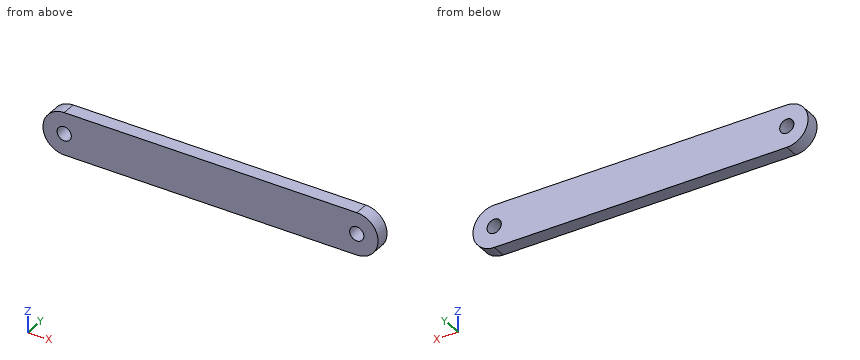
```python
from build123d import *

# Parameters (mm, degrees)
SKETCH1_R           = 2.4
BOSS_EXTRUDE1_DEPTH = 5
SCALE1_SCALE        = 0.8
SKETCH2_R           = 2
CUT_EXTRUDE1_DEPTH  = 48.792424581


with BuildPart() as part:
    # Sketch1 → Boss-Extrude1 (new body)
    with BuildSketch(Plane(origin=(0, 0, 0), x_dir=(1, 0, 0), z_dir=(0, 1, 0))):
        with BuildLine():
            Line((-51.5565916, 7.5), (51.5565916, 7.5))
            ThreePointArc((51.5565916, 7.5), (59.0565916, 0), (51.5565916, -7.5))
            Line((51.5565916, -7.5), (-51.5565916, -7.5))
            ThreePointArc((-51.5565916, -7.5), (-59.0565916, 0), (-51.5565916, 7.5))
        make_face()
        with Locations(Location((-51.5565916, 0, 0), (0, 0, 270))):
            Circle(SKETCH1_R, mode=Mode.SUBTRACT)
        with Locations(Location((51.5565916, 0, 0), (0, 0, 270))):
            Circle(SKETCH1_R, mode=Mode.SUBTRACT)
    extrude(amount=BOSS_EXTRUDE1_DEPTH)


with BuildPart() as part_1:
    # Scale1: scaled about (0, 2.5, 0)
    add(part.part.scale(SCALE1_SCALE).moved(Location((0, 0.5, 0))))

    # Sketch2 → Cut-Extrude1 (cut, through all)
    with BuildSketch(Plane(origin=(0, 4.5, 0), x_dir=(1, 0, 0), z_dir=(0, 1, 0))):
        with Locations(Location((-41.24527328, 0, 0), (0, 0, 270))):
            Circle(SKETCH2_R)
        with Locations(Location((41.24527328, 0, 0), (0, 0, 270))):
            Circle(SKETCH2_R)
    extrude(amount=-CUT_EXTRUDE1_DEPTH, mode=Mode.SUBTRACT)


solid = part_1.part
```
Design review of the part built by this model. Coordinates are the model's own, in mm. Round coordinates to 2 decimals unless told otherwise and drop trailing zeros. Order: outer loops, then holes, each group sorted by start corner. A loop starts at its lowest first (then second) coordinate and runs counter-clockwise, first axis right, second up. Notation, with made-up numbers: (49.25, -32) - (84.25, -32) arc R26 cw to (84.25, -16) - close; hole circle Ø4 at (3, -27). An arc over 180 degrees is marked (long way). Return JSON: item names as keys, results as strings.
Q1. Consider section B-B on y = 1.1. Write out the cut boundary in (x, z), plus the area to 3 significant figures.
Computed values:
{"outline": "(-41.25, -6) - (41.25, -6) arc R6 ccw to (41.25, 6) - (-41.25, 6) arc R6 ccw to start; hole circle Ø4 at (-41.25, 0); hole circle Ø4 at (41.25, 0)", "area": "1,080 mm2"}
Q2. Consider section D-D on z = -4.5. Write out the cut boundary in (x, y), plus the area to 3 significant figures.
Computed values:
{"outline": "(-45.21, 0.5) - (45.21, 0.5) - (45.21, 4.5) - (-45.21, 4.5) - close", "area": "362 mm2"}
Q3. For pin 1 Ø2.5 at (x, z) = (-41.25, 0) entering from -Y, flat-tipped, find the tip position at first contact; note if it passes through.
Computed values:
{"pin 1": "passes through"}
Q4. Consider section C-C on z = 4. Write out the cut boundary in (x, y).
Computed values:
{"outline": "(-45.72, 0.5) - (45.72, 0.5) - (45.72, 4.5) - (-45.72, 4.5) - close"}
Q5. Wall thickness on L1, parallel to X at y = 2.3, z = 0; L2, parallel to X at y = 1.15, z = -0.5; L3, parallel to Z at x = 39.5, y = 2.45: over which ranges is each line inside the solid? List them lowest first. Write a range as [from, to].
Computed values:
{"L1": "x = [-47.25, -43.25], [-39.25, 39.25], [43.25, 47.25]", "L2": "x = [-47.22, -43.18], [-39.31, 39.31], [43.18, 47.22]", "L3": "z = [-6, -0.98], [0.98, 6]"}
Q6. Consider section A-A on z = 0. Write out the cut boundary in (x, y), plus the area to 3 significant figures.
Computed values:
{"outline": "(-47.25, 0.5) - (-43.25, 0.5) - (-43.25, 4.5) - (-47.25, 4.5) - close; (-39.25, 0.5) - (39.25, 0.5) - (39.25, 4.5) - (-39.25, 4.5) - close; (43.25, 0.5) - (47.25, 0.5) - (47.25, 4.5) - (43.25, 4.5) - close", "area": "346 mm2"}
